For this review, take the finished solid that the model builds, in its own axes (mm). A direction names the side the tool comes from. Coordinates: 2 decimals unless noted, no trailing zeros. Order: outer loops, then holes, each group sorted by start corner. A loop starts at its lowest first (then second) coordinate and runs counter-clockwise, first axis right, second up. Notation, with made-up numbers: (21.25, 52) -> (53.25, 52) arc R17 ccw to (53.25, 59) -> close; hole circle Ø11 at (-31, -1). An arc over 180 degrees is marked (long way). Write item = value, one per line. Start each with the question number.
1) Consider section C-C on z = -11.5. Give the boundary of the cut face in (x, y).
2) Insertion check: pin 1 Ø1 at (x, y) = (15.5, 11.5) entering from -Z; pin 2 Ø3 at (y, z) = (8.5, -9) entering from +X; pin 3 Ø2 at (y, z) = (7, -19) entering from +X. Each pin has a flat end and moves straight along its axis. Give the tip position at first contact, or say it passes through.
3) Consider section A-A on x = 26.5. Give the boundary of the cut face in (y, z).
4) Wall thickness on probe 1 along X at (y, z) = (4.5, -9.5); probe 2 along Z at (x, y) = (6, 3.25); probe 3 along X at (y, z) = (8.5, -18.5): over which ranges is each line inside the solid? List them lowest first. Write a range as [from, to].
5) Draft analysis for pull direction Y (two halves, no side actions). For faces 4 (the face through (11, 0, -10)), 5 (the face through (20, 7, -11)), 6 (the face through (12, 15, -10)), 7 (the face through (30, 1, -16)), state which applies: +Y half, -Y half, draft (parallel to the pull), parting line (faces both ways), or undercut.
6) Consider section D-D on y = 13.25. Give the boundary of the cut face in (x, z), and give its area (3 significant figures).
7) Machinability: for faces 1 (the face through (27, 14, -20)), 2 (the face through (25, 1, -19)), 3 (the face through (25, 12.5, -14)), which of the approach directions +Z, -Z, +X, -X, +Y, -Y give a long, thin tool a straight path to every point of the face, cutting with its end or side? Answer none if there is none.
8) Consider section B-B on y = 3.5. Give the boundary of the cut face in (x, z).
from build123d import *

# Parameters (mm, degrees)
F0_W     = 12.5
F0_H     = 15
F1_DEPTH = 20
F2_DEPTH = 20
F4_DEPTH = 15.001
F3_W     = 20
F3_H     = 2.5
F5_DEPTH = 15.001


with BuildPart() as f1:
    # F0 (on Top) → F1 (new body)
    with BuildSketch(Plane.XY):
        with Locations((6.25, 7.5)):
            Rectangle(F0_W, F0_H)
    extrude(amount=-F1_DEPTH)

    # F0 (on Top) → F2 (join)
    with BuildSketch(Plane.XY):
        Polygon((12.5, 15), (12.5, 0), (20, 0), (30, 0), (30, 2.5), (20, 2.5), (20, 12.5), (30, 12.5), (30, 15), (20, 15), align=None)
    extrude(amount=-F2_DEPTH)

    # F3 (on face) → F4 (cut, through all)
    with BuildSketch(Plane.XZ):
        Polygon((30, 0), (12.5, 0), (30, -12.5), align=None)
    extrude(amount=-F4_DEPTH, mode=Mode.SUBTRACT)

    # F3 (on face) → F5 (cut, through all)
    with BuildSketch(Plane.XZ):
        with Locations((15, -18.75)):
            Rectangle(F3_W, F3_H)
    extrude(amount=-F5_DEPTH, mode=Mode.SUBTRACT)


solid = f1.part
Answer sheet:
q1.outline = (0, 0) -> (28.6, 0) -> (28.6, 2.5) -> (20, 2.5) -> (20, 12.5) -> (28.6, 12.5) -> (28.6, 15) -> (0, 15) -> close
q2.pin_1 = -17.5
q2.pin_2 = 20
q2.pin_3 = 5
q3.outline = (0, -20) -> (2.5, -20) -> (2.5, -10) -> (0, -10) -> close; (12.5, -20) -> (15, -20) -> (15, -10) -> (12.5, -10) -> close
q4.probe_1 = [0, 20]
q4.probe_2 = [-17.5, 0]
q4.probe_3 = [0, 5]
q5.face_4 = -Y half
q5.face_5 = undercut
q5.face_6 = +Y half
q5.face_7 = draft
q6.outline = (0, -20) -> (5, -20) -> (5, -17.5) -> (25, -17.5) -> (25, -20) -> (30, -20) -> (30, -12.5) -> (12.5, 0) -> (0, 0) -> close
q6.area = 441 mm2
q7.face_1 = -Z, +X, -X, +Y, -Y
q7.face_2 = -Z, +Y, -Y
q7.face_3 = +Z, -Z, +X
q8.outline = (0, -20) -> (5, -20) -> (5, -17.5) -> (20, -17.5) -> (20, -5.36) -> (12.5, 0) -> (0, 0) -> close
